from build123d import *

# Parameters (mm, degrees)
SKETCH1_R                           = 4
BOSS_EXTRUDE1_DEPTH                 = 195
CUT_EXTRUDE1_REACH                  = 197.082
CUT_EXTRUDE1_END_RADIUS             = 4
SKETCH2_W                           = 1.5
SKETCH2_H                           = 20
CUT_EXTRUDE1_DIRECTION_2_REACH      = 197.082
CUT_EXTRUDE1_DIRECTION_2_END_RADIUS = 4


with BuildPart() as part:
    # Sketch1 → Boss-Extrude1 (new body)
    with BuildSketch(Plane(origin=(0, 0, 0), x_dir=(1, 0, 0), z_dir=(0, 1, 0))):
        with Locations(Location((0, 0, 0), (0, 0, 270))):
            Circle(SKETCH1_R)
    extrude(amount=BOSS_EXTRUDE1_DEPTH)

    # Cut-Extrude1: up to this cylinder (the profile starts inside it)
    cut_extrude1_end = Plane(origin=(0, 97.5, 0), z_dir=(0, -1, 0)) * Cylinder(CUT_EXTRUDE1_END_RADIUS, 578.164, mode=Mode.PRIVATE)
    # Sketch2 → Cut-Extrude1 (cut, up to the surface)
    with BuildSketch(Plane.XY, mode=Mode.PRIVATE) as cut_extrude1_sk1:
        with Locations((3.25, 185)):
            Rectangle(SKETCH2_W, SKETCH2_H)
    cut_extrude1_tool1 = extrude(cut_extrude1_sk1.sketch, amount=-CUT_EXTRUDE1_REACH, mode=Mode.PRIVATE) & cut_extrude1_end
    add(cut_extrude1_tool1.solids().sort_by_distance((3.25, 185, 0))[0], mode=Mode.SUBTRACT)
    # Sketch2 → Cut-Extrude1 (cut, up to the surface)
    with BuildSketch(Plane.XY, mode=Mode.PRIVATE) as cut_extrude1_sk2:
        with Locations((3.25, 142)):
            Rectangle(SKETCH2_W, SKETCH2_H)
    cut_extrude1_tool2 = extrude(cut_extrude1_sk2.sketch, amount=-CUT_EXTRUDE1_REACH, mode=Mode.PRIVATE) & cut_extrude1_end
    add(cut_extrude1_tool2.solids().sort_by_distance((3.25, 142, 0))[0], mode=Mode.SUBTRACT)
    # Sketch2 → Cut-Extrude1 (cut, up to the surface)
    with BuildSketch(Plane.XY, mode=Mode.PRIVATE) as cut_extrude1_sk3:
        with Locations((3.25, 53)):
            Rectangle(SKETCH2_W, SKETCH2_H)
    cut_extrude1_tool3 = extrude(cut_extrude1_sk3.sketch, amount=-CUT_EXTRUDE1_REACH, mode=Mode.PRIVATE) & cut_extrude1_end
    add(cut_extrude1_tool3.solids().sort_by_distance((3.25, 53, 0))[0], mode=Mode.SUBTRACT)
    # Sketch2 → Cut-Extrude1 (cut, up to the surface)
    with BuildSketch(Plane.XY, mode=Mode.PRIVATE) as cut_extrude1_sk4:
        with Locations((3.25, 10)):
            Rectangle(SKETCH2_W, SKETCH2_H)
    cut_extrude1_tool4 = extrude(cut_extrude1_sk4.sketch, amount=-CUT_EXTRUDE1_REACH, mode=Mode.PRIVATE) & cut_extrude1_end
    add(cut_extrude1_tool4.solids().sort_by_distance((3.25, 10, 0))[0], mode=Mode.SUBTRACT)

    # Cut-Extrude1 direction 2: up to this cylinder (the profile starts inside it)
    cut_extrude1_direction_2_end = Plane(origin=(0, 97.5, 0), z_dir=(0, -1, 0)) * Cylinder(CUT_EXTRUDE1_DIRECTION_2_END_RADIUS, 578.164, mode=Mode.PRIVATE)
    # Sketch2 → Cut-Extrude1 direction 2 (cut, up to the surface)
    with BuildSketch(Plane.XY, mode=Mode.PRIVATE) as cut_extrude1_direction_2_sk1:
        with Locations((3.25, 185)):
            Rectangle(SKETCH2_W, SKETCH2_H)
    cut_extrude1_direction_2_tool1 = extrude(cut_extrude1_direction_2_sk1.sketch, amount=CUT_EXTRUDE1_DIRECTION_2_REACH, mode=Mode.PRIVATE) & cut_extrude1_direction_2_end
    add(cut_extrude1_direction_2_tool1.solids().sort_by_distance((3.25, 185, 0))[0], mode=Mode.SUBTRACT)
    # Sketch2 → Cut-Extrude1 direction 2 (cut, up to the surface)
    with BuildSketch(Plane.XY, mode=Mode.PRIVATE) as cut_extrude1_direction_2_sk2:
        with Locations((3.25, 142)):
            Rectangle(SKETCH2_W, SKETCH2_H)
    cut_extrude1_direction_2_tool2 = extrude(cut_extrude1_direction_2_sk2.sketch, amount=CUT_EXTRUDE1_DIRECTION_2_REACH, mode=Mode.PRIVATE) & cut_extrude1_direction_2_end
    add(cut_extrude1_direction_2_tool2.solids().sort_by_distance((3.25, 142, 0))[0], mode=Mode.SUBTRACT)
    # Sketch2 → Cut-Extrude1 direction 2 (cut, up to the surface)
    with BuildSketch(Plane.XY, mode=Mode.PRIVATE) as cut_extrude1_direction_2_sk3:
        with Locations((3.25, 53)):
            Rectangle(SKETCH2_W, SKETCH2_H)
    cut_extrude1_direction_2_tool3 = extrude(cut_extrude1_direction_2_sk3.sketch, amount=CUT_EXTRUDE1_DIRECTION_2_REACH, mode=Mode.PRIVATE) & cut_extrude1_direction_2_end
    add(cut_extrude1_direction_2_tool3.solids().sort_by_distance((3.25, 53, 0))[0], mode=Mode.SUBTRACT)
    # Sketch2 → Cut-Extrude1 direction 2 (cut, up to the surface)
    with BuildSketch(Plane.XY, mode=Mode.PRIVATE) as cut_extrude1_direction_2_sk4:
        with Locations((3.25, 10)):
            Rectangle(SKETCH2_W, SKETCH2_H)
    cut_extrude1_direction_2_tool4 = extrude(cut_extrude1_direction_2_sk4.sketch, amount=CUT_EXTRUDE1_DIRECTION_2_REACH, mode=Mode.PRIVATE) & cut_extrude1_direction_2_end
    add(cut_extrude1_direction_2_tool4.solids().sort_by_distance((3.25, 10, 0))[0], mode=Mode.SUBTRACT)


solid = part.part
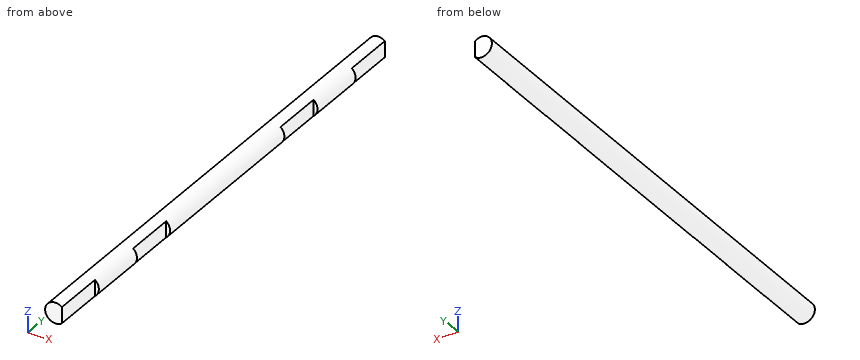
Can you work these out from the model? Positions are in its coordinate system, mm. Coordinates: 2 decimals unless noted, no trailing zeros. Loops run counter-clockwise (first coordinate to the right, second up) from the corner with the lowest first, then second, coordinate; pieces in that order, holes last. Notation, with made-up numbers: (63.25, 33.25) - (91.25, 33.25) arc R11 ccw to (91.25, 54.25) - close; hole circle Ø3 at (-37.5, 1). An arc over 180 degrees is marked (long way). Put each result on its own line as item: value. Start each with the question number.
Item 1: Suppose I cut it at A-A (z = 0). Please give me the cut outline in (x, y).
Item 2: For pin 1 (0.8 mm diameter, centred on x = 3.5, z = 0, fed in from -Y); pin 2 (2 mm diameter, centred on y = 133, z = -2, fed in from -X); pin 3 (1.9 mm diameter, centred on y = 143.5, z = -0.5, fed in from +X), each with a flat end and sliding along its axis, tell me the tip position at first contact or that it passes through.
Item 3: Suppose I cut it at D-D (y = 116). Please give me the cut outline in (x, z).
Item 4: If I drill on line 1 along Y through (x, z) = (2.75, 0); line 2 along X through (y, z) = (155, -2.5); line 3 along X through (y, z) = (55.5, -0.5), over which ranges is the centre line in solid material (lowest first)?
Item 5: Suppose I cut it at B-B (y = 138). Please give me the cut outline in (x, z), and give its area (3 significant figures).
Item 6: Suppose I cut it at C-C (x = -2.25). Please give me the cut outline in (y, z), and give its area (3 significant figures).
Here are the results:
1. outline: (-4, 0) - (2.5, 0) - (2.5, 20) - (4, 20) - (4, 43) - (2.5, 43) - (2.5, 63) - (4, 63) - (4, 132) - (2.5, 132) - (2.5, 152) - (4, 152) - (4, 175) - (2.5, 175) - (2.5, 195) - (-4, 195) - close
2. pin 1: y = 20
2. pin 2: x = -3.87
2. pin 3: x = 2.5
3. outline: circle Ø8 at (0, 0)
4. line 1: 20 to 43, 63 to 132, 152 to 175
4. line 2: -3.12 to 3.12
4. line 3: -3.97 to 2.5
5. outline: (2.5, -3.12) - (2.5, 3.12) arc R4 ccw (long way) to start
5. area: 43.7 mm²
6. outline: (0, -3.31) - (195, -3.31) - (195, 3.31) - (0, 3.31) - close
6. area: 1,290 mm²
